Could you check a few things on this model? Use its own coordinates, in mm. Face numbers are marked on the shaded views. A direction names the side the tool comes from. Coordinates: 2 decimals unless noted, no trailing zeros. Loops run counter-clockwise (first coordinate to the right, second up) from the corner with the lowest first, then second, coordinate; pieces in that order, holes last. Notation, with made-up numbers: M 43,45 L 60,45 A13 cw 60,49 Z; hole C 69,-8 d4. An arc over 180 degrees is marked long. Write each question's results on one line, items separated by ' | '.
```python
from build123d import *

# Parameters (mm, degrees)
F0_W      = 88.9
F0_H      = 38.1
F1_DEPTH  = 50.8
F2_W      = 31.75
F2_H      = 25.4
F3_DEPTH  = 50.8
F4_W      = 25.4
F4_H      = 6.35
F5_DEPTH  = 50.8
F6_W      = 6.35
F6_H      = 25.4
F7_DEPTH  = 50.8
F8_W      = 25.4
F8_H      = 12.7
F9_DEPTH  = 50.8
F10_R     = 6.35
F11_DEPTH = 50.8


with BuildPart() as f1:
    # F0 (on Front) → F1 (new body)
    with BuildSketch(Plane.XZ):
        Rectangle(F0_W, F0_H)
    extrude(amount=F1_DEPTH)

    # F2 (on face) → F3 (cut)
    with BuildSketch(Plane.XZ.offset(50.8)):
        with Locations((28.575, 6.35)):
            Rectangle(F2_W, F2_H)
    extrude(amount=-F3_DEPTH, mode=Mode.SUBTRACT)

    # F4 (on face) → F5 (cut)
    with BuildSketch(Plane.XZ.offset(50.8)):
        with Locations((-12.7, 15.875)):
            Rectangle(F4_W, F4_H)
    extrude(amount=-F5_DEPTH, mode=Mode.SUBTRACT)

    # F6 (on face) → F7 (cut)
    with BuildSketch(Plane.XZ.offset(50.8)):
        with Locations((-41.275, 6.35)):
            Rectangle(F6_W, F6_H)
    extrude(amount=-F7_DEPTH, mode=Mode.SUBTRACT)

    # F8 (on face) → F9 (cut)
    with BuildSketch(Plane.YZ.offset(12.7)):
        with Locations((-25.4, 12.7)):
            Rectangle(F8_W, F8_H)
    extrude(amount=-F9_DEPTH, mode=Mode.SUBTRACT)

    # F10 (on face) → F11 (cut)
    with BuildSketch(Plane.XZ.offset(50.8)):
        with Locations((-6.35, -6.35)):
            Circle(F10_R)
    extrude(amount=-F11_DEPTH, mode=Mode.SUBTRACT)


solid = f1.part
```
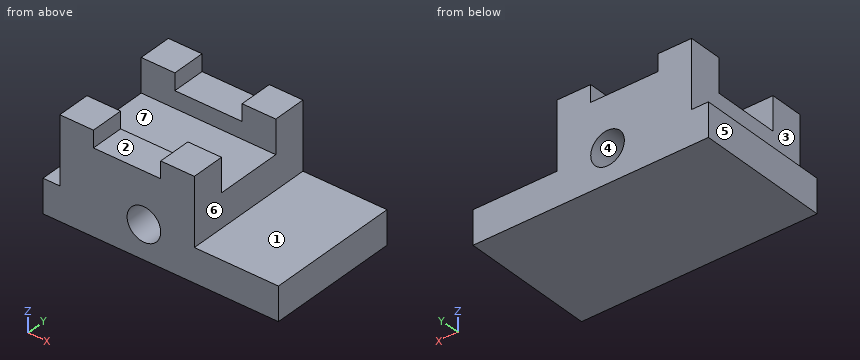
(1) If we mould it in two halves opening along X, with no side actions, what happens to the marked faces 4, 5, 6 and 7? For each: released by +X, released by -X, zero draft, split by the parting line, or undercut.
Reported:
face 4: undercut | face 5: released by -X | face 6: released by +X | face 7: zero draft
(2) Imagine slicing it at A-A, the plane x = -6.35. List the corners of the cut face in (y, z) for me, and give its area (3 significant figures).
Reported:
outline: M -50.8,-19.05 L 0,-19.05 L 0,-12.7 L -50.8,-12.7 Z; M -50.8,0 L 0,0 L 0,12.7 L -12.7,12.7 L -12.7,6.35 L -38.1,6.35 L -38.1,12.7 L -50.8,12.7 Z | area: 806 mm2
(3) Which directions (+Z, -Z, +X, -X, +Y, -Y) give clear straight access to the entire face, cutting with the end or side of a thin tool? Please do the marked faces 1, 2 and 3.
Reported:
face 1: +Z, +X, +Y, -Y | face 2: +Z, +Y, -Y | face 3: +Z, -X, +Y, -Y
(4) Imagine slicing it at C-C, the plane x = -28. List the corners of the cut face in (y, z) for me, and give its area (3 significant figures).
Reported:
outline: M -50.8,-19.05 L 0,-19.05 L 0,19.05 L -12.7,19.05 L -12.7,6.35 L -38.1,6.35 L -38.1,19.05 L -50.8,19.05 Z | area: 1,610 mm2
(5) Imagine slicing it at B-B, the plane y = -17. List the corners of the cut face in (x, z) for me.
Reported:
outline: M -44.45,-19.05 L 44.45,-19.05 L 44.45,-6.35 L 12.7,-6.35 L 12.7,6.35 L -38.1,6.35 L -38.1,-6.35 L -44.45,-6.35 Z; hole C -6.35,-6.35 d12.7
(6) Please list where these lines run through material, in increasing order: probe 1 along Z at (x, y) = (-6.35, -24.5); probe 2 along X at (y, z) = (-23.5, -6); probe 3 along Z at (x, y) = (-6.35, -11). Write a range as from..to.
Reported:
probe 1: z = -19.05..-12.7, 0..6.35 | probe 2: x = -38.1..-12.69, -0.01..12.7 | probe 3: z = -19.05..-12.7, 0..12.7
(7) Imagine slicing it at D-D, the plane y = -8.5. List the corners of the cut face in (x, z) for me, and give its area (3 significant figures).
Reported:
outline: M -44.45,-19.05 L 44.45,-19.05 L 44.45,-6.35 L 12.7,-6.35 L 12.7,19.05 L 0,19.05 L 0,12.7 L -25.4,12.7 L -25.4,19.05 L -38.1,19.05 L -38.1,-6.35 L -44.45,-6.35 Z; hole C -6.35,-6.35 d12.7 | area: 2,130 mm2
(8) Will these pins go through, and if not, where does the flat tip stop? P1, Ø4, axis at x = -16, y = -47, coming from the +Z side; P2, Ø12.5, axis at x = -24, y = -26, coming from the +Z side; P3, Ø7, axis at y = -8.5, z = 15.5, coming from the -X side; P4, Ø7.5, axis at x = -6.35, z = -6.35, coming from the -Y side.
Reported:
P1: stops at z = 12.7 | P2: stops at z = 6.35 | P3: stops at x = -38.1 | P4: passes through
